Autodesk Inventor part; units mm, degrees
ref_plane "YZ Plane" through (0, 0, 0) normal (1, 0, 0) x (0, 1, 0)
ref_plane "XZ Plane" through (0, 0, 0) normal (0, 1, 0) x (-1, 0, 0)
ref_plane "XY Plane" through (0, 0, 0) normal (0, 0, 1) x (1, 0, 0)
sketch "Sketch1" plane through (0, 0, 0) normal (0, 0, 1) x (1, 0, 0)
  line L0 (5, 0) -> (20, 0)
  line L1 (20, 0) -> (20, 15)
  line L2 (15, 20) -> (0, 20)
  line L3 (0, 20) -> (0, 5)
  arc A0 (20, 15) -> (15, 20) centre (15, 15) ccw
  arc A1 (0, 5) -> (5, 0) centre (5, 5) ccw
  point P0 (0, 0)
  point P1 (20, 20)
  dimension "d0" = 20
  dimension "d1" = 20
  dimension "d4" = 5
  dimension "d5" = 5
extrude "Extrusion1" add sketch "Sketch1" along normal blind 22
sketch "Sketch2" plane through (0, 0, 22) normal (0, 0, 1) x (1, 0, 0)
  line L0 (15, 20) -> (0, 20)
  line L1 (20, 0) -> (20, 15)
  point P0 (0, 0)
  point P1 (13.5, 13.5)
  dimension "d13" = 6.5
  dimension "d14" = 6.5
hole "Hole1" at (13.5, 13.5, 22) direction (0, 0, -1) diameter 10 depth 16
sketch "Sketch3" plane through (13.5, 13.5, 6) normal (0, 0, 1) x (1, 0, 0)
  line L0 (6.5, -13.5) -> (6.5, 1.5)
  line L1 (1.5, 6.5) -> (-13.5, 6.5)
  point P0 (-13.5, -13.5)
  point P1 (0, 0)
  dimension "d22" = 6.5
  dimension "d23" = 6.5
hole "Hole2" at (13.5, 13.5, 6) direction (0, 0, -1) diameter 3 depth 16
sketch "Sketch4" plane through (0, 0, 22) normal (0, 0, 1) x (1, 0, 0)
  circle A0 centre (6.5, 6.5) radius 3
  line L0 (5, 0) -> (20, 0)
  line L1 (0, 20) -> (0, 5)
  point P0 (0, 0)
  dimension "d24" = 6
  dimension "d25" = 6.5
  dimension "d26" = 6.5
extrude "Extrusion2" add sketch "Sketch4" along normal blind 5
properties part number "spacer dubbele hoogte behuizing zonder magneet"
Work out the finished part from the listing and answer in its coordinate system (mm). A direction names the side the tool comes from. Coordinates: 2 decimals unless noted, no trailing zeros. Write each loop counter-clockwise with the first axis right and the second up, starting at its lowest first coordinate (ties: lowest second). Pieces come first, ordered by that corner, then holes.
Q1. Which of the six approach directions +Z, -Z, +X, -X, +Y, -Y give full straight-line access (tool end or side, diameter ignored) to faces 1 (the face through (20, 7, 11)), 2 (the face through (15, 15, 6))?
Q2. A cutting plane is placed at A-A, the plane z = 3.75. Give the vertices of the cut face in (x, y).
Q3. This flat-tipped pin is pushed along its axis until it touches: pin 1 Ø11 at (x, y) = (15.5, 14) entering from +Z. Where does it stop, or does it pass through?
Q4. Find the intervals of material crossed by line 1 (X direction, y = 13.5, z = 4.3); line 2 (Y direction, x = 13.5, z = 14.5), in increasing order.
Q5. A cutting plane is placed at D-D, the plane x = 6.5. Give the vertices of the cut face in (y, z), then the cut area to 3 significant figures.
Q6. Determine the mould class of faces 3 (the face through (18, 19, 11)), 4 (the face through (12, 8.73, 13.89)), 5 (the face through (0, 13, 11)) for opening direction X: released by +X, released by -X, zero draft, split by the parting line, or undercut.
Q7. A cutting plane is placed at B-B, the plane x = 13.5. Give the vertices of the cut face in (y, z), then the cut area to 3 significant figures.
Findings below:
1. face 1: +Z, -Z, +X, +Y, -Y
1. face 2: +Z
2. outline: (0, 5) arc R5 ccw to (5, 0) - (20, 0) - (20, 15) arc R5 ccw to (15, 20) - (0, 20) - close; hole circle Ø3 at (13.5, 13.5)
3. pin 1: stops at z = 22
4. line 1: x = 0 to 12, 15 to 20
4. line 2: y = 0 to 8.5, 18.5 to 20
5. outline: (0, 0) - (20, 0) - (20, 22) - (9.5, 22) - (9.5, 27) - (3.5, 27) - (3.5, 22) - (0, 22) - close
5. area: 470 mm2
6. face 3: released by +X
6. face 4: undercut
6. face 5: released by -X
7. outline: (0, 0) - (12, 0) - (12, 6) - (8.5, 6) - (8.5, 22) - (0, 22) - close; (15, 0) - (20, 0) - (20, 22) - (18.5, 22) - (18.5, 6) - (15, 6) - close
7. area: 262 mm2
